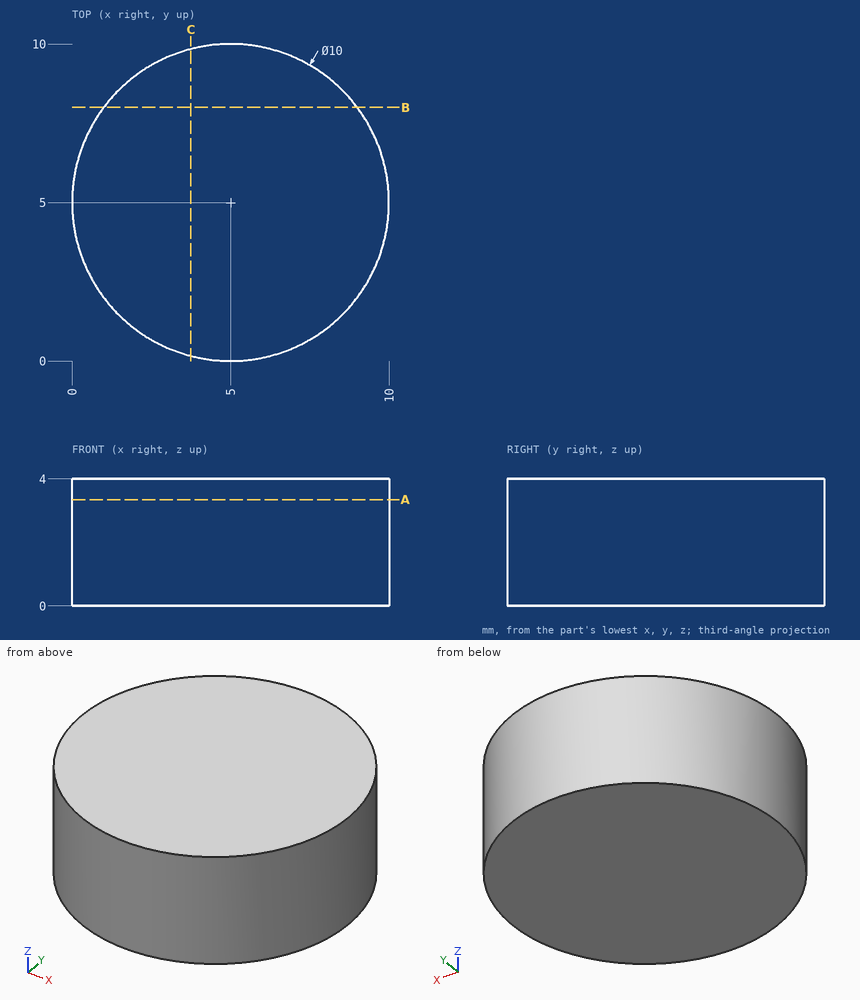
Input: dimensioned drawing with shaded views. Units: mm. Origin: part minimum x, y, z. Coordinates: 2 decimals unless noted, no trailing zeros. Loops run counter-clockwise (first coordinate to the right, second up) from the corner with the lowest first, then second, coordinate; pieces in that order, holes last. Notation, with made-up numbers: M 77.5,-38 L 117.5,-38 A16 cw 117.5,-31 Z; hole C 33.5,36 d2. An arc over 180 degrees is marked long. Use a Markdown table: item, result. Add a question column.
1) Section A-A, the plane z = 3.35. Return the cut outline in (x, y).
2) Section C-C, the plane x = 3.75. Return the cut outline in (y, z), plus the area to 3 significant figures.
3) Line query: L1, parallel to Y at x = 9.25, z = 3.85; L2, parallel to Y at x = 2.75, z = 3.05; L3, parallel to X at y = 4.25, z = 3.55. Output: solid intervals per line, ascending. Write a range as from..to.
4) Section B-B, the plane y = 8. Return the cut outline in (x, z), plus the area to 3 significant figures.
5) Pin query (flat end, axial travel): P1, Ø1, axis at x = 1, z = 3.5, coming from the -Y side; P2, Ø1.5, axis at y = 5.5, z = 1, coming from the +X side; P3, Ø1.5, axis at x = 2.5, z = 1, coming from the +Y side. Return the tip coordinate at first contact, or that it passes through.
Answer below:
| question | item | result |
|---|---|---|
| 1 | outline | C 5,5 d10 |
| 2 | outline | M 0.16,0 L 9.84,0 L 9.84,4 L 0.16,4 Z |
| 2 | area | 38.7 mm2 |
| 3 | L1 | 2.37..7.63 |
| 3 | L2 | 0.53..9.47 |
| 3 | L3 | 0.06..9.94 |
| 4 | outline | M 1,0 L 9,0 L 9,4 L 1,4 Z |
| 4 | area | 32.0 mm2 |
| 5 | P1 | y = 1.43 |
| 5 | P2 | x = 10 |
| 5 | P3 | y = 9.68 |
